Check sheet for the drawn part. Datum: minimum x, y, z corner. Units: mm. A direction names the side the tool comes from. Coordinates: 2 decimals unless noted, no trailing zeros. Order: outer loops, then holes, each group sorted by start corner. A loop starts at its lowest first (then second) coordinate and runs counter-clockwise, first axis right, second up. Notation, with made-up numbers: M 65.5,78 L 108.5,78 A18 ccw 108.5,112 Z; hole C 63.25,84 d3. An arc over 180 degrees is marked long. Return JSON: item names as keys, results as strings. Group by question number.
Q1. Section check D-D, the plane y = 23. Enter the section's corners in (x, z).
Q2. Mould release check, pull along Z, two halves, no side actions. Record for the marked faces 1, 2 and 3: pulls with the +Z half, pulls with the -Z half, needs draft (parallel to the pull), parting line crosses it, or undercut.
Q3. Section check A-A, the plane x = 10.5. Enter the section's corners in (y, z) (1 decimal), then the cut area to 3 significant figures.
Q4. Go/stop test with flat-tipped pins: pin 1 Ø6 at (x, y) = (11, 23.5) entering from -Z; pin 2 Ø2 at (x, z) = (21.5, 6) entering from +Y (1 decimal); pin 3 Ø8 at (x, z) = (7, 12.5) entering from -Y. Record where each tip stops, or that it passes through.
Q5. Thickness scan on probe 1 along Y at (x, z) = (11.5, 16.7); probe 2 along Y at (x, z) = (11.25, 19) (1 decimal); probe 3 along Z at (x, y) = (21.5, 15) (1 decimal). Record the ranges inside material, lowest first.
Q6. Access from +Z, -Z, +X, -X, +Y, -Y to the whole of each face (thin tool, end or side, straight path). Record for the marked faces 4, 5 and 6.
Q7. Section check C-C, the plane y = 15. Enter the section's corners in (x, z) (1 decimal), then the cut area to 3 significant figures.
Q8. Section check B-B, the plane z = 15. Enter the section's corners in (x, y) (1 decimal).
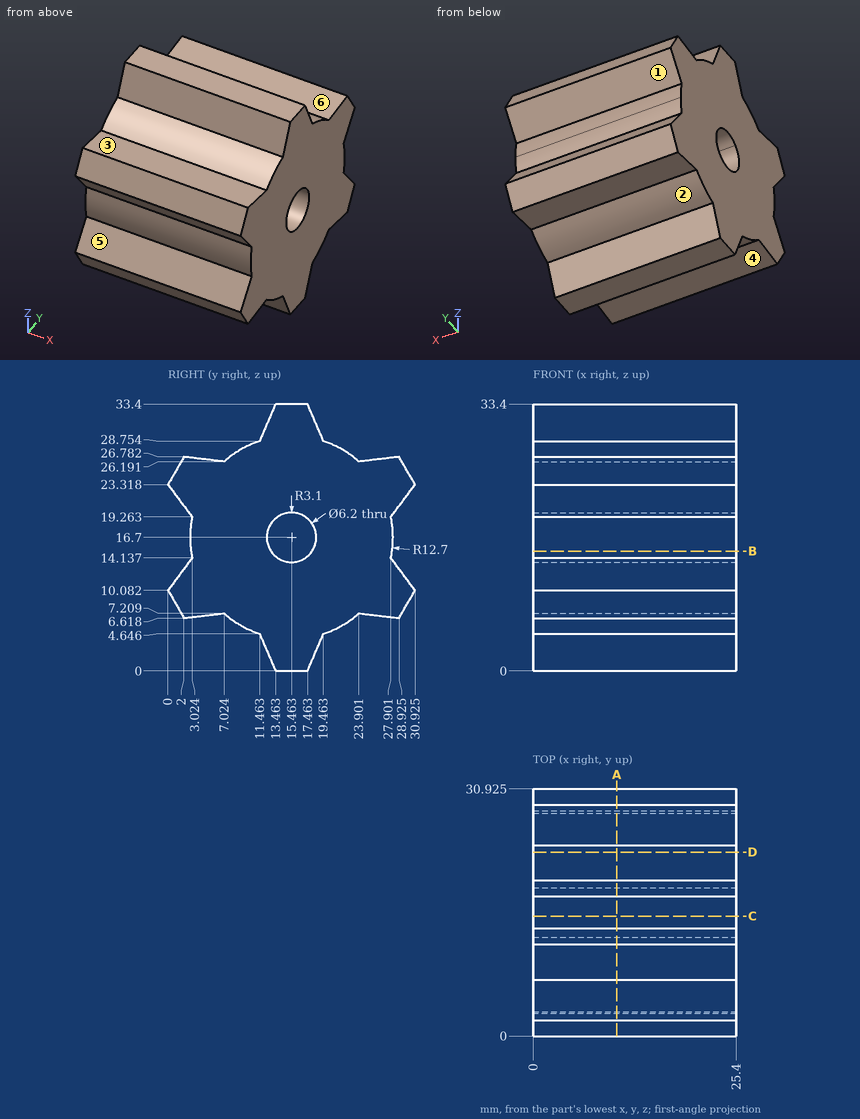
Numbers:
{
 "1": {"outline": "M 0,6.48 L 25.4,6.48 L 25.4,26.92 L 0,26.92 Z"},
 "2": {"face 1": "undercut", "face 2": "pulls with the -Z half", "face 3": "pulls with the +Z half"},
 "3": {"outline": "M 0,10.1 L 2,6.6 L 7,7.2 A12.7 ccw 11.5,4.6 L 13.5,0 L 17.5,0 L 19.5,4.6 A12.7 ccw 23.9,7.2 L 28.9,6.6 L 30.9,10.1 L 27.9,14.1 A12.7 ccw 28.2,16.7 A12.7 ccw 27.9,19.3 L 30.9,23.3 L 28.9,26.8 L 23.9,26.2 A12.7 ccw 19.5,28.8 L 17.5,33.4 L 13.5,33.4 L 11.5,28.8 A12.7 ccw 7,26.2 L 2,26.8 L 0,23.3 L 3,19.3 A12.7 ccw 3,14.1 Z; hole M 13.4,19 A3.1 ccw long 17.5,19 A3.1 ccw Z", "area": "623 mm2"},
 "4": {"pin 1": "stops at z = 5.04", "pin 2": "stops at y = 29.1", "pin 3": "stops at y = 0"},
 "5": {"probe 1": "y = 2.76 to 12.36, 18.56 to 28.16", "probe 2": "y = 3 to 13.4, 17.5 to 28", "probe 3": "z = 0 to 13.6, 19.8 to 33.4"},
 "6": {"face 4": "-Z, +X, -X", "face 5": "+X, -X, -Y", "face 6": "+Z, +X, -X"},
 "7": {"outline": "M 0,0 L 25.4,0 L 25.4,13.6 L 0,13.6 Z; M 0,19.8 L 25.4,19.8 L 25.4,33.4 L 0,33.4 Z", "area": "693 mm2"},
 "8": {"outline": "M 0,2.9 L 25.4,2.9 L 25.4,12.9 L 0,12.9 Z; M 0,18.1 L 25.4,18.1 L 25.4,28 L 0,28 Z"}
}
